from build123d import *

# Parameters (mm, degrees)
F0_W     = 200
F0_H     = 40
F1_DEPTH = 10
F3_DEPTH = 7
F4_R     = 4
F4_R_2   = 3
F4_R_3   = 2.25
F4_R_4   = 1.75
F4_R_5   = 3.25
F4_R_6   = 2.5
F5_DEPTH = 10.001
F6_W     = 15
F6_H     = 47
F6_R     = 2
F7_DEPTH = 10


with BuildPart() as f1:
    # F0 (on Top) → F1 (new body)
    with BuildSketch(Plane.XY):
        Rectangle(F0_W, F0_H)
    extrude(amount=F1_DEPTH)

    # F2 (on face) → F3 (cut)
    with BuildSketch(Plane.XY.offset(10)):
        Polygon((-92.5, -7.794229), (-79, -15.588457), (-65.5, -7.794229), (-65.5, 7.794229), (-79, 15.588457), (-92.5, 7.794229), align=None)
        Polygon((97, -6.928203), (97, 6.928203), (85, 13.856406), (73, 6.928203), (73, -6.928203), (85, -13.856406), align=None)
        Polygon((-56, 6.928203), (-56, -6.928203), (-44, -13.856406), (-32, -6.928203), (-32, 6.928203), (-44, 13.856406), align=None)
        Polygon((50, -15.588457), (63.5, -7.794229), (63.5, 7.794229), (50, 15.588457), (36.5, 7.794229), (36.5, -7.794229), align=None)
        Polygon((-12, 13.856406), (-24, 6.928203), (-24, -6.928203), (-12, -13.856406), (0, -6.928203), (0, 6.928203), align=None)
        Polygon((25, -5.773503), (25, 5.773503), (15, 11.547005), (5, 5.773503), (5, -5.773503), (15, -11.547005), align=None)
    extrude(amount=-F3_DEPTH, mode=Mode.SUBTRACT)

    # F4 (on face) → F5 (cut, through all)
    with BuildSketch(Plane.XY.offset(10)):
        with Locations((-79, 0)):
            Circle(F4_R)
        with Locations((-44, 0)):
            Circle(F4_R_2)
        with Locations((-12, 0)):
            Circle(F4_R_3)
        with Locations((15, 0)):
            Circle(F4_R_4)
        with Locations((50, 0)):
            Circle(F4_R_5)
        with Locations((85, 0)):
            Circle(F4_R_6)
    extrude(amount=-F5_DEPTH, mode=Mode.SUBTRACT)

    # F6 (on face) → F7 (join, through all)
    with BuildSketch(Plane.XY.offset(10)):
        with Locations((60, 43.5)):
            Rectangle(F6_W, F6_H)
        with Locations((60, 60)):
            Circle(F6_R, mode=Mode.SUBTRACT)
        with Locations((-60, 43.5)):
            Rectangle(F6_W, F6_H)
        with BuildLine():
            ThreePointArc((-57.5, 62), (-55.5, 60), (-57.5, 58))
            Line((-57.5, 58), (-62.5, 58))
            ThreePointArc((-62.5, 58), (-64.5, 60), (-62.5, 62))
            Line((-62.5, 62), (-57.5, 62))
        make_face(mode=Mode.SUBTRACT)
    extrude(amount=-F7_DEPTH)


solid = f1.part
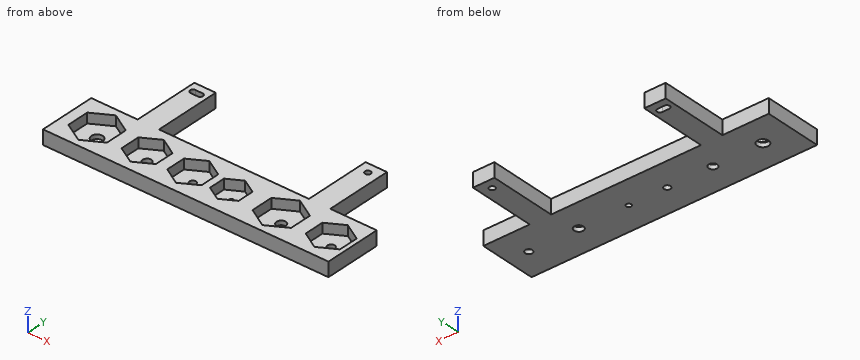
Part model, mm, in its own coordinate system. Give positions to 0.01 mm unless a question says otherwise; leave off trailing zeros. Order: outer loops, then holes, each group sorted by start corner. A loop starts at its lowest first (then second) coordinate and runs counter-clockwise, first axis right, second up. Notation, with made-up numbers: (-1, 13) - (32, 13) arc R33 cw to (32, 52) - close; hole circle Ø10 at (33, 81). An arc over 180 degrees is marked (long way). Use a Markdown table: item, result.
1) Saw through at D-D on y = 0. Count the separate pieces of the cut face and the enclosed holes in it, plus the area to 4 significant figures.
Checked values:
| item | result |
|---|---|
| separate pieces | 7 |
| enclosed holes | 0 |
| area | 877.5 mm² |
2) Saw through at B-B on x = 60. List the corners of the cut face in (y, z), plus the area to 3 significant figures.
Checked values:
| item | result |
|---|---|
| outline | (-20, 0) - (58, 0) - (58, 10) - (9.81, 10) - (9.81, 3) - (-9.81, 3) - (-9.81, 10) - (-20, 10) - close; (62, 0) - (67, 0) - (67, 10) - (62, 10) - close |
| area | 693 mm² |
3) Saw through at A-A on y = 60. List the corners of the cut face in (x, z), plus the area to 3 significant figures.
Checked values:
| item | result |
|---|---|
| outline | (-67.5, 0) - (-64.5, 0) - (-64.5, 10) - (-67.5, 10) - close; (-55.5, 0) - (-52.5, 0) - (-52.5, 10) - (-55.5, 10) - close; (52.5, 0) - (58, 0) - (58, 10) - (52.5, 10) - close; (62, 0) - (67.5, 0) - (67.5, 10) - (62, 10) - close |
| area | 170 mm² |
4) Flat gauge pins, fed straight in: P1, Ø4, axis at x = -74.5, z = 4, coming from the +Y side; P2, Ø2, axis at y = 24.5, z = 1.5, coming from the +X side; P3, Ø13.5, axis at x = 44.5, y = 0.5, coming from the +Z side. Where does each tip first touch, or does it go through?
Checked values:
| item | result |
|---|---|
| P1 | y = 20 |
| P2 | x = 67.5 |
| P3 | z = 3 |
5) Probe L1, parallel to X at y = 57.5, z = 5; L2, parallel to Y at x = -79, z = 0.7; L3, parallel to Y at x = 50, z = 1.15. List the from-to ranges inside material, lowest first. Write a range as from..to.
Checked values:
| item | result |
|---|---|
| L1 | -67.5..-52.5, 52.5..67.5 |
| L2 | -20..-4, 4..20 |
| L3 | -20..-3.25, 3.25..20 |
6) Saw through at C-C on x = 8.5. List the corners of the cut face in (y, z), plus the area to 3 significant figures.
Checked values:
| item | result |
|---|---|
| outline | (-20, 0) - (20, 0) - (20, 10) - (7.79, 10) - (7.79, 3) - (-7.79, 3) - (-7.79, 10) - (-20, 10) - close |
| area | 291 mm² |
